Job drawing, mm, ordinate dimensions from the low corner. One solid piece. A direction names the side the tool comes from. Round coordinates to 2 decimals unless told otherwise and drop trailing zeros. Loops run counter-clockwise (first coordinate to the right, second up) from the corner with the lowest first, then second, coordinate; pieces in that order, holes last. Notation, with made-up numbers: M -35.5,74.25 L -10.5,74.25 A10 ccw -10.5,93.25 Z; hole C 42,66 d9. An arc over 180 degrees is marked long. One line per item, written item: value.
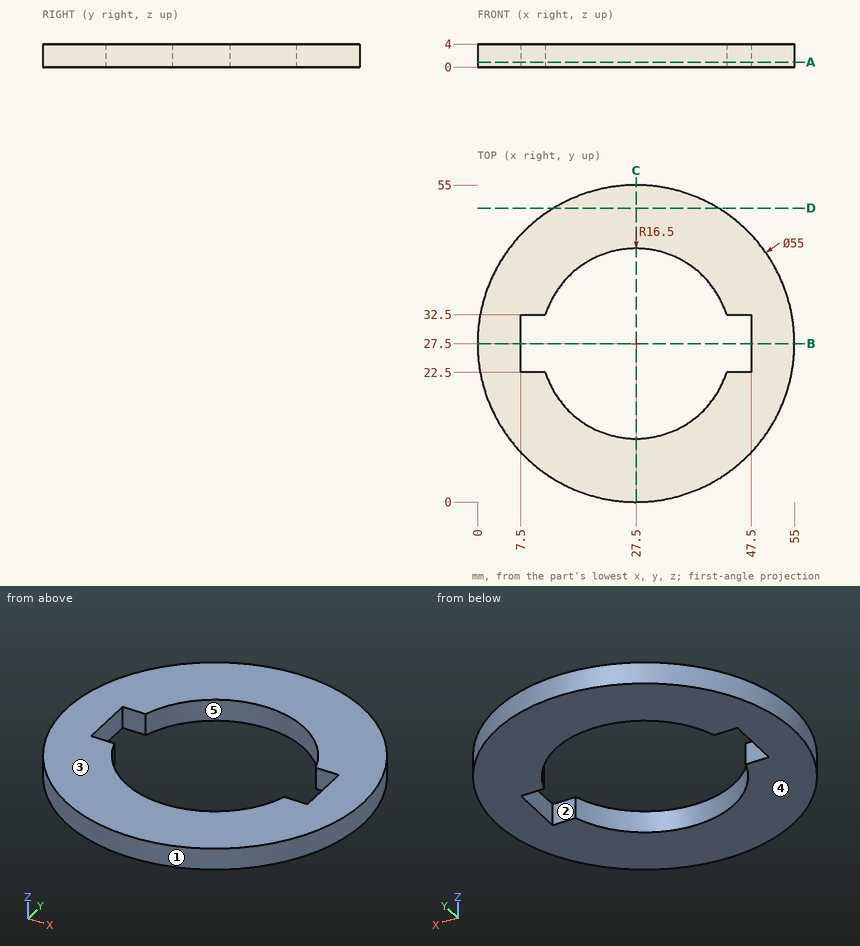
Item 1: Slice it at B-B, the plane y = 27.5. Give the cut face in (x, z), and give its area (3 significant figures).
Check values:
outline: M 0,0 L 7.5,0 L 7.5,4 L 0,4 Z; M 47.5,0 L 55,0 L 55,4 L 47.5,4 Z
area: 60.0 mm2
Item 2: Wall check: line 1 along X through (y, z) = (27, 1.4); line 2 along X through (y, z) = (33.5, 3.5); line 3 along Y through (x, z) = (45, 3.55). Give the ranges that are in metal, low to high.
Check values:
line 1: x = 0 to 7.5, 47.5 to 55
line 2: x = 0.66 to 12.13, 42.87 to 54.34
line 3: y = 6.29 to 22.5, 32.5 to 48.71
Item 3: Slice it at A-A, the plane z = 0.85. Give the cut face in (x, y).
Check values:
outline: C 27.5,27.5 d55; hole M 7.5,22.5 L 11.78,22.5 A16.5 ccw 43.22,22.5 L 47.5,22.5 L 47.5,32.5 L 43.22,32.5 A16.5 ccw 11.78,32.5 L 7.5,32.5 Z
Item 4: Slice it at C-C, the plane x = 27.5. Give the cut face in (y, z).
Check values:
outline: M 0,0 L 11,0 L 11,4 L 0,4 Z; M 44,0 L 55,0 L 55,4 L 44,4 Z
Item 5: Which spindle directions (+Z, -Z, +X, -X, +Y, -Y) get a long thin tool onto all of the face, cutting with end or side? Do the marked faces 4 and 5. Say none if no direction does.
Check values:
face 4: -Z, +X, -X, +Y, -Y
face 5: +Z, -Z
Item 6: Slice it at D-D, the plane y = 51. Give the cut face in (x, z).
Check values:
outline: M 13.22,0 L 41.78,0 L 41.78,4 L 13.22,4 Z
Item 7: Drop flat-ended pins along their axis: P1, Ø2, axis at y = 45.5, z = 1, coming from the -X side; P2, Ø1.2, axis at y = 26.5, z = 2.5, coming from the -X side; P3, Ø2, axis at x = 10.5, z = 1.5, coming from the -Y side. Give the stop position or say it passes through.
Check values:
P1: stops at x = 5.88
P2: stops at x = 0
P3: stops at y = 5.13
Item 8: Pull direction Y, two halves, no side cores. Call the marked faces 1, 2 and 3: pulls with the +Y half, pulls with the -Y half, needs draft (parallel to the pull), parting line crosses it, or undercut.
Check values:
face 1: parting line crosses it
face 2: undercut
face 3: needs draft
